from build123d import *

# Parameters (mm, degrees)
FILLET_1_R = 2


with BuildPart() as part:
    # 草图2 → 旋转1 (revolve)
    with BuildSketch(Plane.XY, mode=Mode.PRIVATE) as revolve_1_sk:
        Polygon((3, 0), (18, 0), (12.5, 23), (0, 23), (0, 0), (0, -40), (3, -40), align=None)
    revolve(revolve_1_sk.sketch.rotate(Axis((0, 0, 0), (0, 1, 0)), 90), axis=Axis((0, 0, 0), (0, 1, 0)))

    # 圆角1
    fillet_1_edges = [part.edges().sort_by_distance(p)[0] for p in [
        (0, 0, 18),
        (0, 23, 12.5),
    ]]
    fillet(fillet_1_edges, radius=FILLET_1_R)


solid = part.part
The listing builds one solid part. Answer for the finished solid, in the listing's coordinates (mm). A direction names the side the tool comes from. Give positions to 0.01 mm unless a question says otherwise; leave off trailing zeros. Loops run counter-clockwise (first coordinate to the right, second up) from the corner with the lowest first, then second, coordinate; pieces in that order, holes last. Notation, with made-up numbers: (-15, 11) - (36, 11) arc R25 ccw to (36, 24) - close; hole circle Ø4 at (1, 48.25). An arc over 180 degrees is marked (long way). Write each question's results on one line, items separated by ' | '.
1. Consider probe 1 along Y at (x, z) = (10, 3); probe 2 along Z at (x, y) = (8, 19.5); probe 3 along X at (y, z) = (12, -11). Determine where each line is inside the solid, lowest interval first. Write a range as from..to.
Resolved:
probe 1: y = 0..23 | probe 2: z = -10.67..10.67 | probe 3: x = -10.39..10.39
2. Find section A-A, the plane z = 0. Write down the section's boundary in (x, y), then the cut area to 3 significant figures.
Resolved:
outline: (-17.41, 2.47) arc R2 ccw to (-15.47, 0) - (-3, 0) - (-3, -40) - (3, -40) - (3, 0) - (15.47, 0) arc R2 ccw to (17.41, 2.47) - (12.87, 21.47) arc R2 ccw to (10.92, 23) - (-10.92, 23) arc R2 ccw to (-12.87, 21.47) - close | area: 938 mm^2
3. Flat-ended cylindrical pins translate along their axes: P1, Ø6, axis at y = 14.5, z = 7, coming from the -X side; P2, Ø6, axis at y = -25, z = -5.5, coming from the -X side; P3, Ø12, axis at y = 11, z = -13.5, coming from the -X side. Find the tip coordinate at first contact, or state that the pin passes through.
Resolved:
P1: stops at x = -14.24 | P2: stops at x = -1.66 | P3: stops at x = -13.79
4. Find section B-B, the plane y = -1. Write down the section's boundary in (x, z), then the cut area to 3 significant figures.
Resolved:
outline: circle Ø6 at (0, 0) | area: 28.3 mm^2
5. Which of the six approach directions +Z, -Z, +X, -X, +Y, -Y give full straight-line access (tool end or side, diameter ignored) to faces 1 (the face through (-0.9, -19.72, -2.86)), 2 (the face through (0, 23, 0))?
Resolved:
face 1: -Y | face 2: +Z, -Z, +X, -X, +Y
6. Find section C-C, the plane y = 17.5. Write down the section's boundary in (x, z).
Resolved:
outline: circle Ø27.63 at (0, 0)
